from build123d import *

# Parameters (mm, degrees)
SKETCH1_W               = 228.6
SKETCH1_H               = 177.8
BOSS_EXTRUDE1_DEPTH     = 9.525
F_1_4_20_TAPPED_HOLE1_D = 6.35
SKETCH5_R               = 35.56
BOSS_EXTRUDE2_DEPTH     = 6.35


with BuildPart() as part:
    # Sketch1 → Boss-Extrude1 (new body)
    with BuildSketch(Plane(origin=(0, 0, 0), x_dir=(1, 0, 0), z_dir=(0, 1, 0))):
        Rectangle(SKETCH1_W, SKETCH1_H)
    extrude(amount=BOSS_EXTRUDE1_DEPTH)

    # 1/4-20 Tapped Hole1 (through all)
    with Locations(Plane(origin=(0, 9.525, 0), x_dir=(-1, 0, 0), z_dir=(0, 1, 0))):
        with Locations((76.2, -57.15), (76.2, 57.15), (-76.2, 57.15), (-76.2, -57.15)):
            Hole(F_1_4_20_TAPPED_HOLE1_D / 2)

    # Sketch5 → Boss-Extrude2 (add)
    with BuildSketch(Plane(origin=(0, 9.525, 0), x_dir=(1, 0, 0), z_dir=(0, 1, 0))):
        with Locations(Location((0, 0, 0), (0, 0, 90))):
            Circle(SKETCH5_R)
    extrude(amount=BOSS_EXTRUDE2_DEPTH)


solid = part.part
Work out the finished part from the listing and answer in its coordinate system (mm). A direction names the side the tool comes from. Coordinates: 2 decimals unless noted, no trailing zeros. Write each loop counter-clockwise with the first axis right and the second up, starting at its lowest first coordinate (ties: lowest second). Pieces come first, ordered by that corner, then holes. Notation, with made-up numbers: M -30,57.5 L 6,57.5 A24 ccw 6,72.5 Z; hole C -18.5,-26 d9. An arc over 180 degrees is marked long. Write item = value, one per line.
1. Flat-ended cylindrical pins translate along their axes: pin 1 (8.5 mm diameter, centred on x = 76.2, z = 57.15, fed in from +Y) (3 decimals); pin 2 (5.5 mm diameter, centred on x = -76.2, z = 57.15, fed in from +Y). Find the tip coordinate at first contact, or state that the pin passes through.
Solution:
pin_1 = 9.525
pin_2 = through
2. The part is cut by section B-B (x = -76.2). Determine the outline of the cut face in (y, z) (3 decimals).
Solution:
outline = M 0,-88.9 L 9.525,-88.9 L 9.525,-60.325 L 0,-60.325 Z; M 0,-53.975 L 9.525,-53.975 L 9.525,53.975 L 0,53.975 Z; M 0,60.325 L 9.525,60.325 L 9.525,88.9 L 0,88.9 Z
3. The part is cut by section C-C (z = 0). Determine the outline of the cut face in (x, y) (3 decimals), then the cut area to 3 significant figures.
Solution:
outline = M -114.3,0 L 114.3,0 L 114.3,9.525 L 35.56,9.525 L 35.56,15.875 L -35.56,15.875 L -35.56,9.525 L -114.3,9.525 Z
area = 2,630 mm2
4. For faces 1 (the face through (-74.735, 4.696, 54.333)), 2 (the face through (-2, 9.525, -41)), determine the directions among +Z, -Z, +X, -X, +Y, -Y from which every point of the face is accessible in a straight line to the end or side of a thin tool.
Solution:
face_1 = +Y, -Y
face_2 = +Y
5. Straight lines are drawn through the part: line 1 (Z direction, x = -76.2, y = 3.75) (3 decimals); line 2 (X direction, y = 1.25, z = -55); line 3 (Y direction, x = -73.5, z = -64.5) (3 decimals). For each, find the intervals that lie inside material, in ascending order. Write a range as from..to.
Solution:
line_1 = -88.9..-60.325, -53.975..53.975, 60.325..88.9
line_2 = -114.3..-78.54, -73.86..73.86, 78.54..114.3
line_3 = 0..9.525
6. Determine the mould class of faces 3 (the face through (34.714, 12.656, 7.709)), 4 (the face through (75.51, 4.7, 54.05)), 5 (the face through (-2, 5, -88.9)) for opening direction X: released by +X, released by -X, zero draft, split by the parting line, or undercut.
Solution:
face_3 = split by the parting line
face_4 = undercut
face_5 = zero draft
7. The part is cut by section A-A (z = 57.15). Determine the outline of the cut face in (x, y) (3 decimals), then the cut area to 3 significant figures.
Solution:
outline = M -114.3,0 L -79.375,0 L -79.375,9.525 L -114.3,9.525 Z; M -73.025,0 L 73.025,0 L 73.025,9.525 L -73.025,9.525 Z; M 79.375,0 L 114.3,0 L 114.3,9.525 L 79.375,9.525 Z
area = 2,060 mm2
8. The part is cut by section D-D (y = 12.75). Determine the outline of the cut face in (x, z).
Solution:
outline = C 0,0 d71.12
